Geometry check sheet. Reference: the model listing, model coordinates, mm. Round coordinates to 2 decimals unless told otherwise and drop trailing zeros. Order: outer loops, then holes, each group sorted by start corner. A loop starts at its lowest first (then second) coordinate and runs counter-clockwise, first axis right, second up.
(1) Go/stop test with flat-tipped pins: pin 1 (5 mm diameter, centred on x = 65, y = 0, fed in from +Z); pin 2 (4 mm diameter, centred on x = -50, y = 0, fed in from +Z). Record where each tip stops, or that it passes through.
(2) Sectioned sample at A-A (x = 1). Record the boundary of the cut face in (y, z), plus the area to 3 significant figures.
(3) Material ranges on line 1 along X through (y, z) = (-0.75, 56); line 2 along Y through (x, z) = (50, 130.5); line 3 along Z through (x, y) = (-0.5, -3.5), recorded low to high.
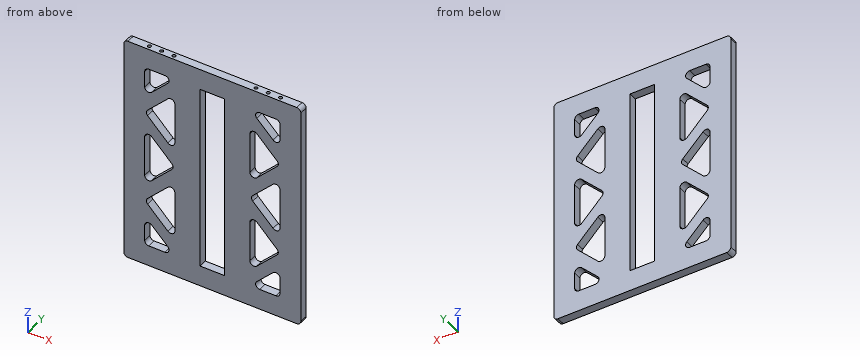
from build123d import *

# Parameters (mm, degrees)
SKETCH1_W                       = 215.9
SKETCH1_H                       = 278
SKETCH1_W_2                     = 30
SKETCH1_H_2                     = 227.2
BOSS_EXTRUDE1_DEPTH             = 5
TAP_DRILL_FOR_M5X0_8_TAP1_D     = 4.2
TAP_DRILL_FOR_M5X0_8_TAP1_DEPTH = 20
TAP_DRILL_FOR_M5X0_8_TAP1_TIP   = 1.2618073
FILLET1_R                       = 5


with BuildPart() as part:
    # Sketch1 → Boss-Extrude1 (new body, symmetric)
    with BuildSketch(Plane(origin=(0, 0, 0), x_dir=(1, 0, 0), z_dir=(0, 1, 0))):
        Rectangle(SKETCH1_W, SKETCH1_H)
        Polygon((-45.75, 113.6), (-82.55, 113.6), (-82.55, 76.8), align=None, mode=Mode.SUBTRACT)
        Rectangle(SKETCH1_W_2, SKETCH1_H_2, mode=Mode.SUBTRACT)
        Polygon((-82.55, 56.8), (-45.75, 93.6), (-45.75, 20), align=None, mode=Mode.SUBTRACT)
        Polygon((-82.55, 36.8), (-45.75, 0), (-82.55, -36.8), align=None, mode=Mode.SUBTRACT)
        Polygon((-82.55, -113.6), (-82.55, -76.8), (-45.75, -113.6), align=None, mode=Mode.SUBTRACT)
        Polygon((-45.75, -93.6), (-45.75, -20), (-82.55, -56.8), align=None, mode=Mode.SUBTRACT)
        Polygon((45.75, -113.6), (82.55, -113.6), (82.55, -76.8), align=None, mode=Mode.SUBTRACT)
        Polygon((82.55, -56.8), (45.75, -93.6), (45.75, -20), align=None, mode=Mode.SUBTRACT)
        Polygon((45.75, 0), (82.55, -36.8), (82.55, 36.8), align=None, mode=Mode.SUBTRACT)
        Polygon((45.75, 93.6), (45.75, 20), (82.55, 56.8), align=None, mode=Mode.SUBTRACT)
        Polygon((82.55, 113.6), (82.55, 76.8), (45.75, 113.6), align=None, mode=Mode.SUBTRACT)
    extrude(amount=BOSS_EXTRUDE1_DEPTH, both=True)

    # Tap Drill for M5x0.8 Tap1
    with Locations(Plane(origin=(-80, 0, 139), x_dir=(1, 0, 0), z_dir=(0, 0, 1))):
        with Locations((0, 0), (15, 0), (30, 0), (130, 0), (145, 0), (160, 0)):
            Hole(TAP_DRILL_FOR_M5X0_8_TAP1_D / 2, depth=TAP_DRILL_FOR_M5X0_8_TAP1_DEPTH)
            with Locations((0, 0, -(TAP_DRILL_FOR_M5X0_8_TAP1_DEPTH + TAP_DRILL_FOR_M5X0_8_TAP1_TIP / 2))):  # 118° drill point
                Cone(0, TAP_DRILL_FOR_M5X0_8_TAP1_D / 2, TAP_DRILL_FOR_M5X0_8_TAP1_TIP, mode=Mode.SUBTRACT)

    # Fillet1
    fillet1_edges = [part.edges().sort_by_distance(p)[0] for p in [
        (45.75, 0, 0),
        (82.55, 0, 36.8),
        (82.55, 0, -56.8),
        (45.75, 0, -93.6),
        (45.75, 0, -20),
        (82.55, 0, -113.6),
        (45.75, 0, -113.6),
        (82.55, 0, -76.8),
        (-82.55, 0, -76.8),
        (-45.75, 0, -113.6),
        (-82.55, 0, -113.6),
        (-82.55, 0, -56.8),
        (-45.75, 0, -20),
        (-45.75, 0, -93.6),
        (-82.55, 0, -36.8),
        (-82.55, 0, 36.8),
        (-45.75, 0, 0),
        (-82.55, 0, 113.6),
        (-45.75, 0, 113.6),
        (-82.55, 0, 76.8),
        (-82.55, 0, 56.8),
        (-45.75, 0, 93.6),
        (-45.75, 0, 20),
        (-107.95, 0, -139),
        (82.55, 0, 76.8),
        (45.75, 0, 113.6),
        (107.95, 0, -139),
        (82.55, 0, 113.6),
        (107.95, 0, 139),
        (-107.95, 0, 139),
        (82.55, 0, 56.8),
        (45.75, 0, 20),
        (45.75, 0, 93.6),
        (82.55, 0, -36.8),
    ]]
    fillet(fillet1_edges, radius=FILLET1_R)


solid = part.part
Answer below:
1. pin 1: stops at z = 139
1. pin 2: stops at z = 118.94
2. outline: (-5, -139) - (5, -139) - (5, -113.6) - (-5, -113.6) - close; (-5, 113.6) - (5, 113.6) - (5, 139) - (-5, 139) - close
2. area: 508 mm2
3. line 1: x = -107.95 to -80.41, -45.75 to -15, 15 to 45.75, 80.41 to 107.95
3. line 2: y = -5 to -2.1, 2.1 to 5
3. line 3: z = -139 to -113.6, 113.6 to 139
